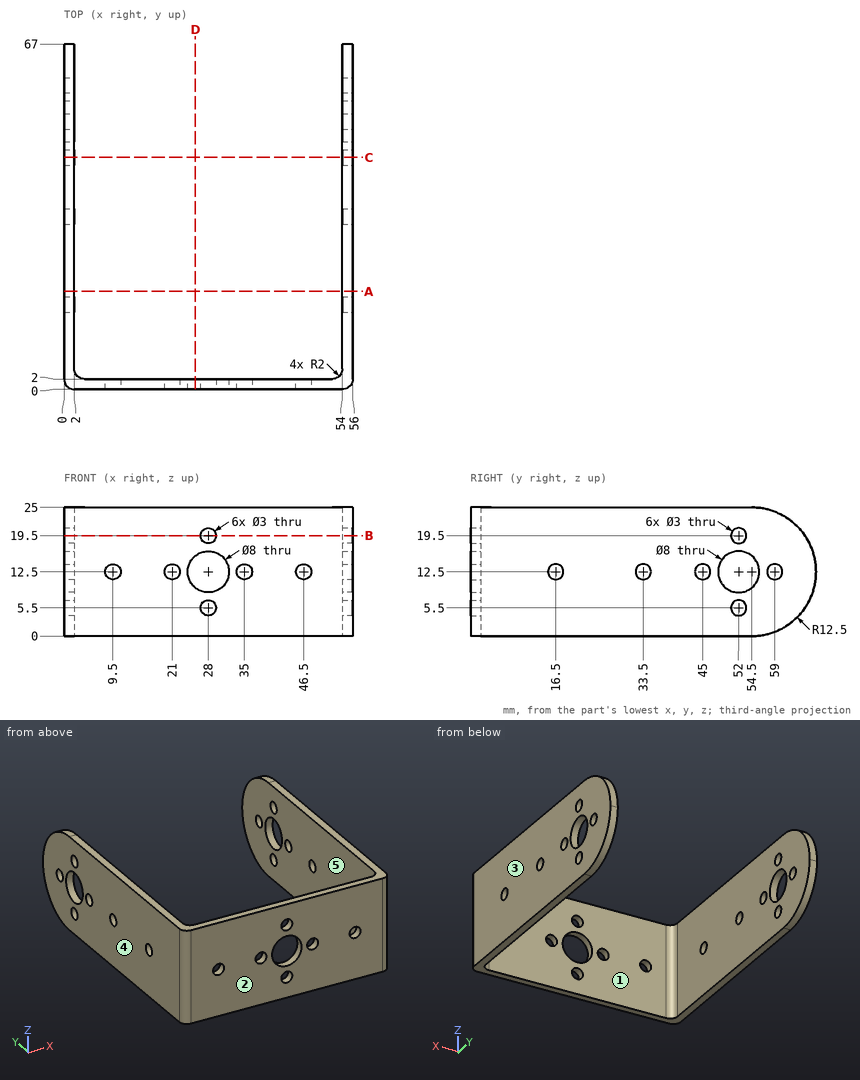
Verification items for this drawing (mm, ordinates from the low corner). A direction names the side the tool comes from. Coordinates: 2 decimals unless noted, no trailing zeros. Write each loop counter-clockwise with the first axis right and the second up, starting at its lowest first coordinate (ties: lowest second). Pieces come first, ordered by that corner, then holes. Notation, with made-up numbers: M -6,15.5 L 47,15.5 A22 cw 47,33.5 Z; hole C -38,24 d2. An arc over 180 degrees is marked long. One line per item, written item: value. Start each with the question number.
(1) Tool access check on the marked faces 1 and 2. Record the directions out of +Z, -Z, +X, -X, +Y, -Y that give a thin tool (end or side, any length) a straight path to the whole face; none if there is none.
(2) Sectioned sample at C-C, the plane y = 45. Enter the section's corners in (x, z).
(3) Scan lines: line 1 along X through (y, z) = (45, 17.5); line 2 along X through (y, z) = (1.55, 12.5); line 3 along Y through (x, z) = (5.5, 20.75). Record each from-to range of solid material in increasing order. Write a range as [from, to].
(4) Release check for a two-part mould opening along X. For the marked faces 3, 4 and 5 record: released by +X, released by -X, zero draft, split by the parting line, or undercut.
(5) Sectioned sample at A-A, the plane y = 19. Enter the section's corners in (x, z), and give its area (3 significant figures).
(6) Depth check by flat-ended pin: pin 1 (12.5 mm diameter, centred on y = 34.5, z = 11, fed in from -X); pin 2 (2.5 mm diameter, centred on x = 9.5, z = 12.5, fed in from +Y); pin 3 (10 mm diameter, centred on x = 24.5, z = 8, fed in from +Y). Enter the tip coordinate at first touch or a pass-through.
(7) Sectioned sample at B-B, the plane z = 19.5. Enter the section's corners in (x, y).
(8) Sectioned sample at D-D, the plane x = 25.5. Enter the section's corners in (y, z), and give its area (3 significant figures).
Filled sheet:
1. face 1: +Z, -Z, +Y
1. face 2: +Z, -Z, +X, -X, -Y
2. outline: M 0,0 L 2,0 L 2,11 L 0,11 Z; M 0,14 L 2,14 L 2,25 L 0,25 Z; M 54,0 L 56,0 L 56,11 L 54,11 Z; M 54,14 L 56,14 L 56,25 L 54,25 Z
3. line 1: [0, 2], [54, 56]
3. line 2: [0.05, 8], [11, 19.5], [22.5, 24], [32, 33.5], [36.5, 45], [48, 55.95]
3. line 3: [0, 2]
4. face 3: released by +X
4. face 4: released by -X
4. face 5: undercut
5. outline: M 0,0 L 2,0 L 2,25 L 0,25 Z; M 54,0 L 56,0 L 56,25 L 54,25 Z
5. area: 100 mm²
6. pin 1: x = 0
6. pin 2: through
6. pin 3: y = 2
7. outline: M 0,2 A2 ccw 2,0 L 26.5,0 L 26.5,2 L 4,2 A2 cw 2,4 L 2,50.5 L 0,50.5 Z; M 0,53.5 L 2,53.5 L 2,64.86 L 0,64.86 Z; M 29.5,0 L 54,0 A2 ccw 56,2 L 56,50.5 L 54,50.5 L 54,4 A2 cw 52,2 L 29.5,2 Z; M 54,53.5 L 56,53.5 L 56,64.86 L 54,64.86 Z
8. outline: M 0,0 L 2,0 L 2,9.38 L 0,9.38 Z; M 0,15.62 L 2,15.62 L 2,25 L 0,25 Z
8. area: 37.5 mm²
